Design review of the part built by this model. Coordinates are the model's own, in mm. A direction names the side the tool comes from. Coordinates: 2 decimals unless noted, no trailing zeros. Write each loop counter-clockwise with the first axis right and the second up, starting at its lowest first coordinate (ties: lowest second). Pieces come first, ordered by that corner, then holes. Notation, with made-up numbers: (21, 5.5) -> (46, 5.5) arc R18 ccw to (46, 21.5) -> close; hole circle Ø11 at (87, 50.5). An arc over 180 degrees is marked (long way). One line per question, with ' | ' between items. Start each with the question number.
Q1. Add section D-D on z = 0. State the section outline as (x, y) points, and give its area (3 significant figures).
Q2. Add section A-A on y = 13. State the section outline as (x, z) points.
Q3. Wall thickness on probe 1 along X at (y, z) = (5.5, 32); probe 2 along Y at (x, z) = (15.5, 8): over which ranges is each line inside the solid? List them lowest first.
Q4. Add section C-C on y = 6.5. State the section outline as (x, z) points, and give its area (3 significant figures).
Q5. Draft analysis for pull direction Z (two halves, no side actions). For faces 3 (the cylindrical face through (46.99, 7.4, -47.15)), 4 (the flat face through (-1, 7, 50)), 5 (the flat face through (38.111, 12.282, 38.163)), 6 (the flat face through (0, 32, 0)), state which applies: pulls with the +Z half, pulls with the -Z half, needs draft (parallel to the pull), parting line crosses it, or undercut.
Q6. Add section B-B on z = -32. State the section outline as (x, y) points.
Q7. For P1, Ø3.5, axis at x = -32, z = -32, coming from the -Y side; P2, Ø2, axis at x = 16.5, z = 1.5, coming from the +Y side; P3, Ø5, axis at y = 28, z = 9.5, coming from the +X side, all flat-tipped, find the tip position at first contact; note any pin that passes through.
Q8. For faces 1 (the flat face through (-38.29, 14.75, 38.34)), 2 (the cylindrical face through (-35, 5, 32)), list the 3-axis set-ups (+Z, -Z, +X, -X, +Y, -Y) from which the entire face can be reached by the end or side of a thin tool; tool diameter is ignored.
Autodesk Inventor part; units mm, degrees
ref_plane "YZ Plane" through (0, 0, 0) normal (1, 0, 0) x (0, 1, 0)
ref_plane "XZ Plane" through (0, 0, 0) normal (0, 1, 0) x (-1, 0, 0)
ref_plane "XY Plane" through (0, 0, 0) normal (0, 0, 1) x (1, 0, 0)
sketch "Sketch1" plane through (0, 0, 0) normal (0, 1, 0) x (-1, 0, 0)
  line L0 (40, 50) -> (-40, 50)
  line L1 (-50, 40) -> (-50, -40)
  line L2 (-40, -50) -> (40, -50)
  line L3 (50, -40) -> (50, 40)
  line L4 (50, 50) -> (-50, -50) construction
  line L5 (-50, 50) -> (50, -50) construction
  arc A0 (-40, 50) -> (-50, 40) centre (-40, 40) ccw
  arc A1 (50, 40) -> (40, 50) centre (40, 40) ccw
  arc A2 (-50, -40) -> (-40, -50) centre (-40, -40) ccw
  arc A3 (40, -50) -> (50, -40) centre (40, -40) ccw
  point P0 (0, 0)
  dimension "d0" = 100
  dimension "d1" = 100
  dimension "d2" = 10
  dimension "d3" = 10
  dimension "d4" = 10
extrude "Extrusion1" add sketch "Sketch1" along normal blind 15
sketch "Sketch2" plane through (0, 15, 0) normal (0, 1, 0) x (1, 0, 0)
  line L0 (-36.2734, -40) -> (36.2734, -40)
  line L1 (40, -36.2734) -> (40, 36.2734)
  line L2 (36.2734, 40) -> (-36.2734, 40)
  line L3 (-40, 36.2734) -> (-40, -36.2734)
  line L4 (-40, -40) -> (40, 40) construction
  line L5 (40, -40) -> (-40, 40) construction
  line L6 (-36.2734, -40) -> (-40, -36.2734)
  line L7 (-36.2734, 40) -> (-40, 36.2734)
  line L8 (36.2734, -40) -> (40, -36.2734)
  line L9 (36.2734, 40) -> (40, 36.2734)
  point P0 (0, 0)
  dimension "d7" = 80
  dimension "d8" = 80
  dimension "d9" = 3.7266
  dimension "d10" = 3.7266
  dimension "d11" = 3.7266
  dimension "d12" = 3.7266
  dimension "d13" = 3.7266
  dimension "d14" = 3.7266
  dimension "d15" = 3.7266
  dimension "d16" = 3.7266
extrude "Extrusion2" cut sketch "Sketch2" against normal blind 5
sketch "Sketch3" plane through (0, 10, 0) normal (0, 1, 0) x (1, 0, 0)
  line L0 (0, 0) -> (32, 0)
  line L1 (32, 0) -> (32, -32)
  circle A0 centre (32, -32) radius 3
  circle A1 centre (32, 32) radius 3
  circle A2 centre (-32, 32) radius 3
  circle A3 centre (-32, -32) radius 3
  dimension "d19" = 32
  dimension "d20" = 32
  dimension "d21" = 6
  dimension "d24" = 360
  dimension "d44" = 6
extrude "Extrusion3" cut sketch "Sketch3" against normal blind 20
sketch "Sketch4" plane through (0, 10, 0) normal (0, 1, 0) x (1, 0, 0)
  circle A0 centre (0, 0) radius 12
  dimension "d28" = 24
extrude "Extrusion4" add sketch "Sketch4" along normal blind 17
sketch "Sketch5" plane through (0, 27, 0) normal (0, 1, 0) x (1, 0, 0)
  circle A0 centre (0, 0) radius 10
  dimension "d31" = 20
extrude "Extrusion5" add sketch "Sketch5" along normal blind 5
fillet "Fillet1" radius 0.5 2 edges at (-12, 27, 0) (-10, 32, 0)
chamfer "Chamfer1" distance 0.5 angle 45 12 edges at (-35, 10, 32) (29, 10, 32) (29, 10, -32) (-35, 10, -32) (0, 15, 40) (-38.1367, 15, 38.1367) (-40, 15, 0) (-38.1367, 15, -38.1367) (0, 15, -40) (38.1367, 15, -38.1367) (40, 15, 0) (38.1367, 15, 38.1367)
equation "\"d0\" = d1"
equation "\"d8\" = d7"
equation "\"d10\" = d9"
equation "\"d11\" = d9"
equation "\"d12\" = d9"
equation "\"d13\" = d9"
equation "\"d14\" = d9"
equation "\"d15\" = d9"
equation "\"d16\" = d9"
properties part number "Base1"
Output values:
1) outline: (-50, 0) -> (50, 0) -> (50, 15) -> (40.5, 15) -> (40, 14.5) -> (40, 10) -> (12, 10) -> (12, 26.5) arc R0.5 ccw to (11.5, 27) -> (10, 27) -> (10, 31.5) arc R0.5 ccw to (9.5, 32) -> (-9.5, 32) arc R0.5 ccw to (-10, 31.5) -> (-10, 27) -> (-11.5, 27) arc R0.5 ccw to (-12, 26.5) -> (-12, 10) -> (-40, 10) -> (-40, 14.5) -> (-40.5, 15) -> (-50, 15) -> close | area: 1,610 mm2
2) outline: (-50, -40) arc R10 ccw to (-40, -50) -> (40, -50) arc R10 ccw to (50, -40) -> (50, 40) arc R10 ccw to (40, 50) -> (-40, 50) arc R10 ccw to (-50, 40) -> close; circle Ø24 at (0, 0); hole (-40, -36.27) -> (-36.27, -40) -> (36.27, -40) -> (40, -36.27) -> (40, 36.27) -> (36.27, 40) -> (-36.27, 40) -> (-40, 36.27) -> close
3) probe 1: x = -50 to -35, -29 to 29, 35 to 50 | probe 2: y = 0 to 10
4) outline: (-50, -40) arc R10 ccw to (-40, -50) -> (40, -50) arc R10 ccw to (50, -40) -> (50, 40) arc R10 ccw to (40, 50) -> (-40, 50) arc R10 ccw to (-50, 40) -> close; hole circle Ø6 at (-32, -32); hole circle Ø6 at (-32, 32); hole circle Ø6 at (32, -32); hole circle Ø6 at (32, 32) | area: 9,800 mm2
5) face 3: pulls with the -Z half | face 4: pulls with the +Z half | face 5: undercut | face 6: needs draft
6) outline: (-50, 0) -> (-35, 0) -> (-35, 9.5) -> (-35.5, 10) -> (-40, 10) -> (-40, 14.5) -> (-40.5, 15) -> (-50, 15) -> close; (-29, 0) -> (29, 0) -> (29, 9.5) -> (28.5, 10) -> (-28.5, 10) -> (-29, 9.5) -> close; (35, 0) -> (50, 0) -> (50, 15) -> (40.5, 15) -> (40, 14.5) -> (40, 10) -> (35.5, 10) -> (35, 9.5) -> close
7) P1: passes through | P2: stops at y = 10 | P3: stops at x = 9.42
8) face 1: +Y | face 2: +Y, -Y
